Read the model definition and answer for the solid it produces. Units are mm, in the model's axes. A direction names the side the tool comes from. Coordinates: 2 decimals unless noted, no trailing zeros. Order: outer loops, then holes, each group sorted by start corner. A loop starts at its lowest first (then second) coordinate and runs counter-clockwise, first axis right, second up.
```python
from build123d import *

# Parameters (mm, degrees)
BOSS_EXTRUDE1_DEPTH = 20
CUT_EXTRUDE1_DEPTH  = 17
SKETCH4_R           = 25
SKETCH4_R_2         = 20
CUT_EXTRUDE2_DEPTH  = 0.5
FILLET1_R           = 10
FILLET2_R           = 5


with BuildPart() as part:
    # Sketch2 → Boss-Extrude1 (new body)
    with BuildSketch(Plane.XY):
        with BuildLine():
            ThreePointArc((88, 0), (-42.971685161, 76.794754212), (-46.032597146, -75))
            Line((-46.032597146, -75), (46.032597146, -75))
            ThreePointArc((46.032597146, -75), (76.794754212, -42.971685161), (88, 0))
        make_face()
    extrude(amount=-BOSS_EXTRUDE1_DEPTH)

    # Sketch3 → Cut-Extrude1 (cut)
    with BuildSketch(Plane(origin=(0, 0, -20), x_dir=(-1, 0, 0), z_dir=(0, 0, -1))):
        with BuildLine():
            Line((-43.116122275, -65), (43.116122275, -65))
            ThreePointArc((43.116122275, -65), (0, 78), (-43.116122275, -65))
        make_face()
    extrude(amount=-CUT_EXTRUDE1_DEPTH, mode=Mode.SUBTRACT)

    # Sketch4 → Cut-Extrude2 (cut)
    with BuildSketch(Plane.XY):
        with Locations((0, -3)):
            Circle(SKETCH4_R)
        with Locations(Location((-54.77, -38, 0), (0, 0, 180))):
            Circle(SKETCH4_R_2)
        with Locations((35, 51.77)):
            Circle(SKETCH4_R_2)
        with Locations((54.77, -38)):
            Circle(SKETCH4_R_2)
        with Locations(Location((-35, 51.77, 0), (0, 0, 180))):
            Circle(SKETCH4_R_2)
    extrude(amount=-CUT_EXTRUDE2_DEPTH, mode=Mode.SUBTRACT)

    # Fillet1
    fillet1_edges = [part.edges().sort_by_distance(p)[0] for p in [
        (43.116122275, -65, -11.5),
        (-43.116122275, -65, -11.5),
    ]]
    fillet(fillet1_edges, radius=FILLET1_R)

    # Fillet2
    fillet2_edges = [part.edges().sort_by_distance(p)[0] for p in [
        (-46.032597146, -75, -10),
        (46.032597146, -75, -10),
    ]]
    fillet(fillet2_edges, radius=FILLET2_R)


solid = part.part
```
1) Flat-ended cylindrical pins translate along their axes: pin 1 Ø1.5 at (x, y) = (-1.5, -31.5) entering from +Z; pin 2 Ø2 at (x, y) = (-46.5, -18.5) entering from -Z; pin 3 Ø12 at (x, y) = (-50.5, -32) entering from +Z; pin 4 Ø5 at (y, z) = (15, -13) entering from +X. Find the tip coordinate at first contact, or state that the pin passes through.
A:
pin 1: stops at z = 0
pin 2: stops at z = -3
pin 3: stops at z = -0.5
pin 4: stops at x = 87.11
2) A cutting plane is placed at C-C, the plane y = 39. Determine the outline of the cut face in (x, z), and give its area (3 significant figures).
A:
outline: (-78.89, -20) - (-67.55, -20) - (-67.55, -3) - (67.55, -3) - (67.55, -20) - (78.89, -20) - (78.89, 0) - (50.39, 0) - (50.39, -0.5) - (19.61, -0.5) - (19.61, 0) - (-19.61, 0) - (-19.61, -0.5) - (-50.39, -0.5) - (-50.39, 0) - (-78.89, 0) - close
area: 828 mm2
3) A cutting plane is placed at B-B, the plane x = 0. Determine the outline of the cut face in (y, z).
A:
outline: (-75, -20) - (-65, -20) - (-65, -3) - (78, -3) - (78, -20) - (88, -20) - (88, 0) - (22, 0) - (22, -0.5) - (-28, -0.5) - (-28, 0) - (-75, 0) - close
4) Determine the mould class of faces 4 (the flat face through (-1, -75, -10)), 5 (the flat face through (35, 52, -0.5)), 6 (the flat face through (-1, 26, 0)) for opening direction Y: pulls with the +Y half, pulls with the -Y half, needs draft (parallel to the pull), parting line crosses it, or undercut.
A:
face 4: pulls with the -Y half
face 5: undercut
face 6: needs draft
5) Straight lines are drawn through the part: line 1 (Y direction, x = -2, z = -16); line 2 (X direction, y = -2.5, z = -11.5); line 3 (Z direction, x = 8.5, y = 65). For each, find the intervals that lie inside material, in ascending order.
A:
line 1: y = -75 to -65, 77.97 to 87.98
line 2: x = -87.96 to -77.96, 77.96 to 87.96
line 3: z = -3 to 0
6) Which of the six approach directions +Z, -Z, +X, -X, +Y, -Y give full straight-line access (tool end or side, diameter ignored) to faces 1 (the flat face through (0, -3, -0.5)), 2 (the cylindrical face through (-43.121, -64.496, -11.381)), 3 (the flat face through (0, -66, -20))?
A:
face 1: +Z
face 2: -Z
face 3: -Z, +X, -X, +Y, -Y
7) A cutting plane is placed at D-D, the plane y = -24. Determine the outline of the cut face in (x, z), and give its area (3 significant figures).
A:
outline: (-84.66, -20) - (-74.22, -20) - (-74.22, -3) - (74.22, -3) - (74.22, -20) - (84.66, -20) - (84.66, 0) - (69.05, 0) - (69.05, -0.5) - (40.49, -0.5) - (40.49, 0) - (13.56, 0) - (13.56, -0.5) - (-13.56, -0.5) - (-13.56, 0) - (-40.49, 0) - (-40.49, -0.5) - (-69.05, -0.5) - (-69.05, 0) - (-84.66, 0) - close
area: 821 mm2
8) A cutting plane is placed at A-A, the plane z = -13. Determine the outline of the cut face in (x, y), and give its area (3 significant figures).
A:
outline: (-47.28, -74.22) arc R5 ccw to (-44.6, -75) - (44.6, -75) arc R5 ccw to (47.28, -74.22) arc R88 ccw (long way) to start; hole (-45.87, -63.09) arc R10 ccw to (-39.99, -65) - (39.99, -65) arc R10 ccw to (45.87, -63.09) arc R78 ccw (long way) to start
area: 5,170 mm2
